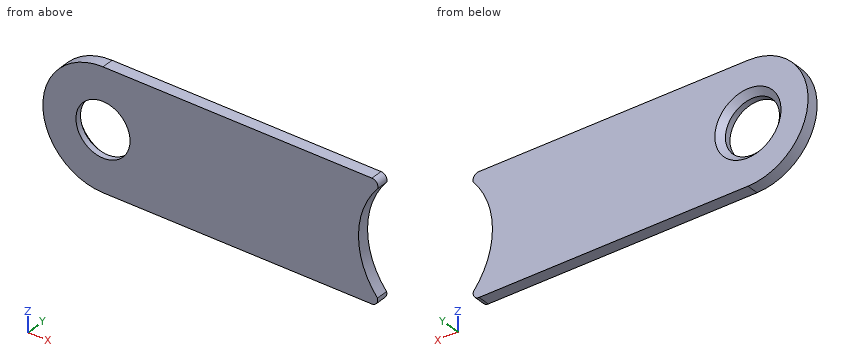
Autodesk Fusion 360 part; units mm, degrees
sketch "Sketch1" plane through (0, 0, 0) normal (0, 1, 0) x (1, 0, 0)
  line L0 (17.4087, -54.8067) -> (135.0065, -54.8067) construction
  circle A0 centre (37.1699, -54.8067) radius 10
  line L1 (9.2396, -44.8067) -> (81.8771, -44.8067) construction
  line L2 (13.4192, -64.8067) -> (138.6161, -64.8067) construction
  circle A1 centre (37.1699, -54.8067) radius 4.5
  circle A2 centre (37.1699, -54.8067) radius 7.5 construction
  line L3 (44.6699, -37.6811) -> (44.6699, -71.7825) construction
  line L4 (46.6699, -36.8465) -> (46.6699, -73.6307) construction
  line L5 (79.6699, -35.9522) -> (79.6699, -73.0345) construction
  line L6 (93.1699, -35.833) -> (93.1699, -73.7499) construction
  circle A3 centre (93.1699, -54.7914) radius 13.5
  line L7 (37.1699, -44.8067) -> (84.084, -44.8067)
  line L8 (37.1699, -64.8067) -> (81.9057, -64.8067)
  line L9 (82.084, -39.2431) -> (82.084, -68.9507) construction
  line L10 (82.6289, -46.466) -> (82.084, -47.0874)
  line L11 (82.6565, -63.1461) -> (82.084, -62.4955)
  arc A4 (82.6289, -46.466) -> (81.8771, -44.8067) centre (81.8771, -45.8067) ccw
  arc A5 (81.9057, -64.8067) -> (82.6565, -63.1461) centre (81.9057, -63.8067) ccw
  dimension "d1" = 20
  dimension "d2" = 9
  dimension "d3" = 15
  dimension "d4" = 2
  dimension "d5" = 33
  dimension "d6" = 13.5
  dimension "d7" = 27
  dimension "d8" = 2
  dimension "d9" = 1
  dimension "d10" = 1
extrude "Extrude1" add sketch "Sketch1" along normal blind 2 contours A0 | A0 A3 L7 L8 A4 A5
chamfer "Chamfer1" distance 1 angle 45 1 edges at (32.9745, 2, 53.1794)
equation "d6 = ( 27 / 2 ) * 1 mm"
Input: part model. Units: mm. Frame: model coordinates. Give positions to 0.01 mm unless a question says otherwise; leave off trailing zeros. Write each loop counter-clockwise with the first axis right and the second up, starting at its lowest first coordinate (ties: lowest second). Pieces come first, ordered by that corner, then holes. Notation, with made-up numbers: (-29, -13.5) -> (-11, -13.5) arc R13 ccw to (-11, -3.5) -> close; hole circle Ø7 at (-30, -21.75). An arc over 180 degrees is marked (long way). Use one line per item in the form item = value. Start each with the question number.
1) Section query B-B on z = 61. Return the cut outline in (x, y), then the cut area to 3 significant figures.
2) Ray query, probe 1 along X at (y, z) = (1.8, 51.5); probe 2 along X at (y, z) = (1.75, 56.25); probe 3 along X at (y, z) = (1.45, 64). Return the intervals inside material, ascending. Write a range as from..to.
3) Section query A-A on y = 1.55. Return the cut outline in (x, z).
Outcome:
q1.outline = (29.32, 0) -> (81.18, 0) -> (81.18, 2) -> (29.32, 2) -> close
q1.area = 104 mm^2
q2.probe_1 = 27.73..33.03, 41.31..80.08
q2.probe_2 = 27.27..32.12, 42.22..79.75
q2.probe_3 = 33.24..82.89
q3.outline = (37.17, 44.81) -> (81.88, 44.81) arc R1 ccw to (82.83, 46.11) arc R13.5 cw to (82.86, 63.51) arc R1 ccw to (81.91, 64.81) -> (37.17, 64.81) arc R10 ccw to start; hole circle Ø10.1 at (37.17, 54.81)
